Design review of the part built by this model. Coordinates are the model's own, in mm. A direction names the side the tool comes from. Give positions to 0.01 mm unless a question says otherwise; leave off trailing zeros. Order: outer loops, then holes, each group sorted by start corner. A loop starts at its lowest first (then second) coordinate and runs counter-clockwise, first axis right, second up. Notation, with made-up numbers: (-30, 58.25) -> (-1, 58.25) arc R34 cw to (-1, 93.25) -> close; hole circle Ø9 at (-3, 10). An arc over 180 degrees is marked (long way). Return JSON: item names as keys, results as strings.
```python
from build123d import *

# Parameters (mm, degrees)
SKETCH_W        = 50
SKETCH_H        = 20
PAD_DEPTH       = 20
SKETCH001_W     = 10
SKETCH001_H     = 16
POCKET_DEPTH    = 16
POCKET001_DEPTH = 30
SKETCH003_R     = 2.4
POCKET002_DEPTH = 4
SKETCH004_R     = 2.4
POCKET003_DEPTH = 4


with BuildPart() as part:
    # Sketch → Pad (new body)
    with BuildSketch(Plane.XY):
        with Locations((25, 10)):
            Rectangle(SKETCH_W, SKETCH_H)
    extrude(amount=PAD_DEPTH)

    # Sketch001 → Pocket (cut)
    with BuildSketch(Plane.XY.offset(20)):
        with Locations((5, 12)):
            Rectangle(SKETCH001_W, SKETCH001_H)
        with Locations((45, 12)):
            Rectangle(SKETCH001_W, SKETCH001_H)
    extrude(amount=-POCKET_DEPTH, mode=Mode.SUBTRACT)

    # Sketch002 → Pocket001 (cut)
    with BuildSketch(Plane.YZ.offset(40)):
        Polygon((20, 4), (4, 20), (20, 20), align=None)
    extrude(amount=-POCKET001_DEPTH, mode=Mode.SUBTRACT)

    # Sketch003 → Pocket002 (cut)
    with BuildSketch(Plane(origin=(0, 4, 0), x_dir=(-1, 0, 0), z_dir=(0, 1, 0))):
        with Locations((-45, 12)):
            Circle(SKETCH003_R)
        with Locations((-5, 12)):
            Circle(SKETCH003_R)
    extrude(amount=-POCKET002_DEPTH, mode=Mode.SUBTRACT)

    # Sketch004 → Pocket003 (cut)
    with BuildSketch(Plane.XY.offset(4)):
        with Locations((5, 12)):
            Circle(SKETCH004_R)
        with Locations((45, 12)):
            Circle(SKETCH004_R)
    extrude(amount=-POCKET003_DEPTH, mode=Mode.SUBTRACT)


solid = part.part
```
Item 1: Add section C-C (x = 5). Give the boundary of the cut face in (y, z), plus the area to 3 significant figures.
Result set:
{"outline": "(0, 0) -> (9.6, 0) -> (9.6, 4) -> (4, 4) -> (4, 9.6) -> (0, 9.6) -> close; (0, 14.4) -> (4, 14.4) -> (4, 20) -> (0, 20) -> close; (14.4, 0) -> (20, 0) -> (20, 4) -> (14.4, 4) -> close", "area": "106 mm^2"}
Item 2: For pin 1 (8 mm diameter, centred on y = 11, z = 13, fed in from -X); pin 2 (3 mm diameter, centred on x = 46, y = 11.5, fed in from +Z); pin 3 (6 mm diameter, centred on x = 45, z = 12, fed in from +Y), all flat-tipped, find the tip position at first contact; note any pin that passes through.
Result set:
{"pin 1": "stops at x = 10", "pin 2": "stops at z = 4", "pin 3": "stops at y = 4"}
Item 3: Wall thickness on L1, parallel to Z at x = 5, y = 2.1; L2, parallel to Y at x = 47, z = 10.25: over which ranges is each line inside the solid? List them lowest first. Write a range as [from, to].
Result set:
{"L1": "z = [0, 9.6], [14.4, 20]", "L2": "y = [0, 4]"}
Item 4: Mouldability with a two-part tool opening along Y and no side actions: class faces 1 (the face through (25, 20, 2)), 2 (the face through (50, 5, 3)), 3 (the face through (42.602, 12.106, 2.028)), 4 (the face through (6.29, 14.024, 2.028)) as released by +Y, released by -Y, zero draft, split by the parting line, or undercut.
Result set:
{"face 1": "released by +Y", "face 2": "zero draft", "face 3": "undercut", "face 4": "undercut"}
Item 5: Add section A-A (z = 12). Give the boundary of the cut face in (x, y), plus the area to 3 significant figures.
Result set:
{"outline": "(0, 0) -> (2.6, 0) -> (2.6, 4) -> (0, 4) -> close; (7.4, 0) -> (42.6, 0) -> (42.6, 4) -> (40, 4) -> (40, 12) -> (10, 12) -> (10, 4) -> (7.4, 4) -> close; (47.4, 0) -> (50, 0) -> (50, 4) -> (47.4, 4) -> close", "area": "402 mm^2"}
Item 6: Add section D-D (z = 7). Give the boundary of the cut face in (x, y).
Result set:
{"outline": "(0, 0) -> (50, 0) -> (50, 4) -> (40, 4) -> (40, 17) -> (10, 17) -> (10, 4) -> (0, 4) -> close"}
Item 7: Machinability: for faces 5 (the face through (47.398, 2.028, 12.106)), 6 (the face through (10, 8, 9)), 7 (the face through (40, 8, 9)), which of the approach directions +Z, -Z, +X, -X, +Y, -Y give a long, thin tool a straight path to every point of the face, cutting with its end or side? Answer none if there is none.
Result set:
{"face 5": "+Y, -Y", "face 6": "+Z, -X, +Y", "face 7": "+Z, +X, +Y"}
